from build123d import *

# Parameters (mm, degrees)
SKETCH1_R                = 1.5
BOSS_EXTRUDE1_DEPTH      = 19
SKETCH2_W                = 3
SKETCH2_H                = 5
BOSS_EXTRUDE2_DEPTH      = 5
SKETCH3_R                = 0.584411026
CUT_EXTRUDE1_DEPTH       = 5
BOSS_EXTRUDE3_DEPTH      = 8
BOSS_EXTRUDE3_DEPTH_BACK = 27
BOSS_EXTRUDE4_DEPTH      = 11
BOSS_EXTRUDE5_DEPTH      = 8.5
BOSS_EXTRUDE6_DEPTH      = 6


with BuildPart() as part:
    # Sketch1 → Boss-Extrude1 (new body)
    with BuildSketch(Plane.XY):
        with BuildLine():
            Line((-18.5, -11), (13.5, -11))
            ThreePointArc((13.5, -11), (17.035533906, -9.535533906), (18.5, -6))
            Line((18.5, -6), (18.5, 6))
            ThreePointArc((18.5, 6), (17.035533906, 9.535533906), (13.5, 11))
            Line((13.5, 11), (-18.5, 11))
            Line((-18.5, 11), (-18.5, -11))
        make_face()
        with Locations((-13.5, 8.5)):
            Circle(SKETCH1_R, mode=Mode.SUBTRACT)
        with Locations((-13.5, -8.5)):
            Circle(SKETCH1_R, mode=Mode.SUBTRACT)
    extrude(amount=BOSS_EXTRUDE1_DEPTH)

    # Sketch2 → Boss-Extrude2 (add)
    with BuildSketch(Plane(origin=(18.5, 0, 0), x_dir=(0, 0, -1), z_dir=(1, 0, 0))):
        with Locations((-9.5, 0)):
            Rectangle(SKETCH2_W, SKETCH2_H)
    extrude(amount=BOSS_EXTRUDE2_DEPTH)

    # Sketch3 → Cut-Extrude1 (cut)
    with BuildSketch(Plane.XY.offset(11)):
        with Locations((21, 0)):
            Circle(SKETCH3_R)
    extrude(amount=-CUT_EXTRUDE1_DEPTH, mode=Mode.SUBTRACT)

    # Sketch4 → Boss-Extrude3 (add, two sides)
    with BuildSketch(Plane.XY.offset(19)) as boss_extrude3_sk:
        with BuildLine():
            Line((8.589724736, 2.25), (8.589724736, -2.25))
            ThreePointArc((8.589724736, -2.25), (7.5, -2.5), (6.410275264, -2.25))
            Line((6.410275264, -2.25), (6.410275264, 2.25))
            ThreePointArc((6.410275264, 2.25), (7.5, 2.5), (8.589724736, 2.25))
        make_face()
    extrude(amount=BOSS_EXTRUDE3_DEPTH)
    extrude(boss_extrude3_sk.sketch, amount=-BOSS_EXTRUDE3_DEPTH_BACK)

    # Sketch5 → Boss-Extrude4 (add)
    with BuildSketch(Plane.ZY.offset(18.5)):
        with BuildLine():
            ThreePointArc((9.500000028, 11), (4.022680904, 9.539338317), (0, 5.545268253))
            Line((0, 5.545268253), (0, -5.545268253))
            ThreePointArc((0, -5.545268253), (4.022680873, -9.539338299), (9.499999955, -11))
            ThreePointArc((9.499999955, -11), (14.977319088, -9.539338321), (19, -5.545268253))
            Line((19, -5.545268253), (19, 5.545268253))
            ThreePointArc((19, 5.545268253), (14.97731912, 9.539338303), (9.500000028, 11))
        make_face()
    extrude(amount=BOSS_EXTRUDE4_DEPTH)

    # Sketch6 → Boss-Extrude5 (add)
    with BuildSketch(Plane.ZY.offset(29.5)):
        with BuildLine():
            Line((1, 5.267826876), (1, -5.267826876))
            ThreePointArc((1, -5.267826876), (9.5, -10), (18, -5.267826876))
            Line((18, -5.267826876), (18, 5.267826876))
            ThreePointArc((18, 5.267826876), (9.5, 10), (1, 5.267826876))
        make_face()
    extrude(amount=BOSS_EXTRUDE5_DEPTH)

    # Sketch7 → Boss-Extrude6 (add)
    with BuildSketch(Plane.ZY.offset(38)):
        with BuildLine():
            ThreePointArc((1, -5.267826876), (9.5, -10), (18, -5.267826876))
            Line((18, -5.267826876), (18, 5.267826876))
            ThreePointArc((18, 5.267826876), (9.5, 10), (1, 5.267826876))
            Line((1, 5.267826876), (1, -5.267826876))
        make_face()
    extrude(amount=BOSS_EXTRUDE6_DEPTH)


solid = part.part
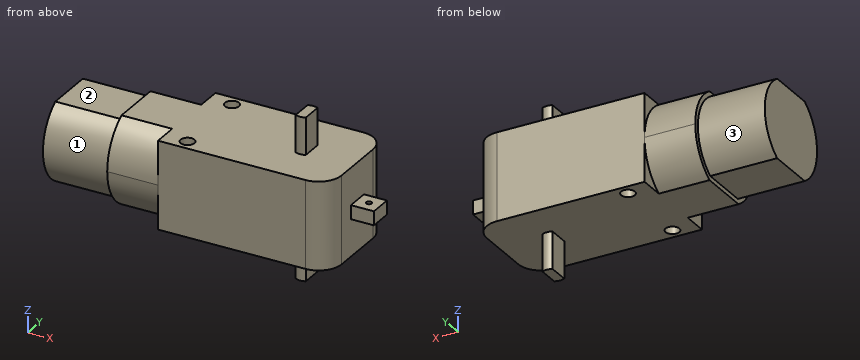
For this review, take the finished solid that the model builds, in its own axes (mm). Face numbers are marked on the shaded views. A direction names the side the tool comes from. Round coordinates to 2 decimals unless told otherwise and drop trailing zeros. Order: outer loops, then holes, each group sorted by start corner. A loop starts at its lowest first (then second) coordinate and runs counter-clockwise, first axis right, second up. Notation, with made-up numbers: (78.25, -2.5) -> (136.25, -2.5) arc R12 cw to (136.25, 5.5) -> close; hole circle Ø10 at (-22.75, 26.5). An arc over 180 degrees is marked (long way). Write item = value, one per line. Start each with the question number.
1) Take a section at A-A on x = -13.5. State the section outline as (y, z) points.
2) Take a section at D-D on y = 8.5. State the section outline as (x, z) points, plus the area to 3 significant figures.
3) Insertion check: pin 1 (1.9 mm diameter, centred on x = 21, y = 0, fed in from -Z); pin 2 (12 mm diameter, centred on x = -16.5, y = -4, fed in from -Z); pin 3 (1 mm diameter, centred on x = -27.5, y = -1, fed in from +Z). Each pin has a flat end and moves straight along its axis. Give the tip position at first contact, or say it passes through.
4) Tool access review of the marked faces 1, 2 and 3: name each direction out of +Z, -Z, +X, -X, +Y, -Y from which nothing blocks a thin tool from reaching the whole face with its end or side.
5) Take a section at B-B on y = -4. State the section outline as (x, z) points, plus the area to 3 significant figures.
6) To check wall thickness, follow line 1 (Y direction, x = 21, z = 9); line 2 (X direction, y = 4, z = 13); line 3 (Z direction, x = 15, y = -7.5). State the ranges of each line that lie inside material, in increasing order. Write a range as from..to.
7) Take a section at C-C on z = 12.5. State the section outline as (x, y) points.
Verdict:
q1.outline = (-11, 0) -> (-10, 0) -> (-10, 19) -> (-11, 19) -> close; (-7, 0) -> (7, 0) -> (7, 19) -> (-7, 19) -> close; (10, 0) -> (11, 0) -> (11, 19) -> (10, 19) -> close
q2.outline = (-44, 4.23) -> (-29.5, 4.23) -> (-29.5, 2.52) -> (-18.5, 2.52) -> (-18.5, 0) -> (-15, 0) -> (-15, 19) -> (-18.5, 19) -> (-18.5, 16.48) -> (-29.5, 16.48) -> (-29.5, 14.77) -> (-44, 14.77) -> close; (-12, 0) -> (17.83, 0) -> (17.83, 19) -> (-12, 19) -> close
q2.area = 940 mm2
q3.pin_1 = 8
q3.pin_2 = 0
q3.pin_3 = 19
q4.face_1 = -X, -Y
q4.face_2 = +Z, -X, +Y, -Y
q4.face_3 = -X, +Y
q5.outline = (-44, 1) -> (-29.5, 1) -> (-29.5, 0) -> (18.5, 0) -> (18.5, 19) -> (-29.5, 19) -> (-29.5, 18) -> (-44, 18) -> close
q5.area = 1,160 mm2
q6.line_1 = -2.5..-0.58, 0.58..2.5
q6.line_2 = -44..18.5
q6.line_3 = 0..19
q7.outline = (-44, -9.54) -> (-29.5, -9.54) -> (-29.5, -10.58) -> (-18.5, -10.58) -> (-18.5, -11) -> (13.5, -11) arc R5 ccw to (18.5, -6) -> (18.5, 6) arc R5 ccw to (13.5, 11) -> (-18.5, 11) -> (-18.5, 10.58) -> (-29.5, 10.58) -> (-29.5, 9.54) -> (-44, 9.54) -> close; hole circle Ø3 at (-13.5, -8.5); hole circle Ø3 at (-13.5, 8.5)
